```python
from build123d import *

# Parameters (mm, degrees)
SKETCH1_R                       = 90
BOSS_EXTRUDE1_DEPTH             = 2
CUT_EXTRUDE1_DEPTH              = 3
SKETCH5_R                       = 1.75
CUT_EXTRUDE3_DEPTH              = 3
MIRROR2_COPY_1_DEPTH            = 3
MIRROR2_COPY_2_SKETCH_R         = 1.75
MIRROR2_COPY_2_DEPTH            = 3
CUT_EXTRUDE2_DEPTH              = 3
SKETCH6_R                       = 10
CUT_EXTRUDE4_DEPTH              = 3
SKETCH7_R                       = 1.75
CUT_EXTRUDE5_DEPTH              = 3
CIRPATTERN1_COUNT               = 4
CIRPATTERN1_ANGLE               = 36
CIRPATTERN1_THE_OTHER_WAY_COUNT = 4
CIRPATTERN1_THE_OTHER_WAY_ANGLE = 36
SKETCH8_R                       = 1.75
CUT_EXTRUDE6_DEPTH              = 3
SKETCH9_R                       = 1.75
CUT_EXTRUDE7_DEPTH              = 3
CIRPATTERN2_COUNT               = 2
CIRPATTERN2_ANGLE               = 8
CIRPATTERN2_THE_OTHER_WAY_COUNT = 2
CIRPATTERN2_THE_OTHER_WAY_ANGLE = 8
MIRROR3_COPY_1_SKETCH_R         = 1.75
MIRROR3_COPY_1_DEPTH            = 3
MIRROR3_COPY_2_SKETCH_R         = 1.75
MIRROR3_COPY_2_DEPTH            = 3
SKETCH10_R                      = 2
CUT_EXTRUDE8_DEPTH              = 3
LPATTERN1_COUNT                 = 5
LPATTERN1_PITCH                 = 10
LPATTERN1_COPY_1_SKETCH_R       = 2
LPATTERN1_COPY_1_DEPTH          = 3
LPATTERN1_COPY_2_SKETCH_R       = 2
LPATTERN1_COPY_2_DEPTH          = 3
LPATTERN1_COPY_3_SKETCH_R       = 2
LPATTERN1_COPY_3_DEPTH          = 3
LPATTERN1_COPY_4_SKETCH_R       = 2
LPATTERN1_COPY_4_DEPTH          = 3


with BuildPart() as part:
    # Sketch1 → Boss-Extrude1 (new body)
    with BuildSketch(Plane(origin=(0, 0, 0), x_dir=(1, 0, 0), z_dir=(0, 1, 0))):
        Circle(SKETCH1_R)
    extrude(amount=BOSS_EXTRUDE1_DEPTH)

    # Sketch3 → Cut-Extrude1 (cut, through all)
    with BuildSketch(Plane(origin=(0, 2, 0), x_dir=(1, 0, 0), z_dir=(0, 1, 0))):
        Polygon((-106.374227687, 31.753350771), (-80.374227687, 76.786671768), (-49.197313151, 58.786671768), (-75.197313151, 13.753350771), align=None)
    cut_extrude1 = extrude(amount=-CUT_EXTRUDE1_DEPTH, mode=Mode.SUBTRACT)

    # Sketch5 → Cut-Extrude3 (cut, through all)
    with BuildSketch(Plane(origin=(0, 2, 0), x_dir=(1, 0, 0), z_dir=(0, 1, 0))):
        with Locations((-60.537059113, 19.145655616)):
            Circle(SKETCH5_R)
        with Locations((-46.537059113, 43.394366922)):
            Circle(SKETCH5_R)
    cut_extrude3 = extrude(amount=-CUT_EXTRUDE3_DEPTH, mode=Mode.SUBTRACT)

    # Mirror1: Cut-Extrude1, Cut-Extrude3 across plane
    add(cut_extrude1.mirror(Plane.XY), mode=Mode.SUBTRACT)
    add(cut_extrude3.mirror(Plane.XY), mode=Mode.SUBTRACT)

    # Mirror2: Cut-Extrude1, Cut-Extrude3 across plane
    add(cut_extrude1.mirror(Plane(origin=(0, 0, 0), x_dir=(0, 0, 1), z_dir=(1, 0, 0))), mode=Mode.SUBTRACT)
    add(cut_extrude3.mirror(Plane(origin=(0, 0, 0), x_dir=(0, 0, 1), z_dir=(1, 0, 0))), mode=Mode.SUBTRACT)

    # Mirror2 copy 1 sketch → Mirror2 copy 1 (cut, through all)
    with BuildSketch(Plane(origin=(0, 2, 0), x_dir=(-1, 0, 0), z_dir=(0, 1, 0))):
        Polygon((-106.374227687, 31.753350771), (-80.374227687, 76.786671768), (-49.197313151, 58.786671768), (-75.197313151, 13.753350771), align=None)
    extrude(amount=-MIRROR2_COPY_1_DEPTH, mode=Mode.SUBTRACT)

    # Mirror2 copy 2 sketch → Mirror2 copy 2 (cut, through all)
    with BuildSketch(Plane(origin=(0, 2, 0), x_dir=(-1, 0, 0), z_dir=(0, 1, 0))):
        with Locations((-60.537059113, 19.145655616)):
            Circle(MIRROR2_COPY_2_SKETCH_R)
        with Locations((-46.537059113, 43.394366922)):
            Circle(MIRROR2_COPY_2_SKETCH_R)
    extrude(amount=-MIRROR2_COPY_2_DEPTH, mode=Mode.SUBTRACT)

    # Sketch4 → Cut-Extrude2 (cut, through all)
    with BuildSketch(Plane(origin=(0, 2, 0), x_dir=(1, 0, 0), z_dir=(0, 1, 0))):
        with BuildLine():
            Line((-42.5, 79.333158263), (-42.5, 69.333158263))
            ThreePointArc((-42.5, 69.333158263), (0, 55), (42.5, 69.333158263))
            Line((42.5, 69.333158263), (42.5, 79.333158263))
            Line((42.5, 79.333158263), (42.5, 105.809765059))
            Line((42.5, 105.809765059), (-42.5, 105.809765059))
            Line((-42.5, 105.809765059), (-42.5, 79.333158263))
        make_face()
    extrude(amount=-CUT_EXTRUDE2_DEPTH, mode=Mode.SUBTRACT)

    # Sketch6 → Cut-Extrude4 (cut, through all)
    with BuildSketch(Plane(origin=(0, 2, 0), x_dir=(1, 0, 0), z_dir=(0, 1, 0))):
        Circle(SKETCH6_R)
    extrude(amount=-CUT_EXTRUDE4_DEPTH, mode=Mode.SUBTRACT)

    # Sketch7 → Cut-Extrude5 (cut, through all)
    with BuildSketch(Plane.XZ):
        with Locations((0, 86)):
            Circle(SKETCH7_R)
    cut_extrude5 = extrude(amount=-CUT_EXTRUDE5_DEPTH, mode=Mode.SUBTRACT)

    # CirPattern1: Cut-Extrude5 ×4 about axis
    cirpattern1_axis = Axis((0, 0, 0), (0, 1, 0))
    for i in range(1, CIRPATTERN1_COUNT):
        add(cut_extrude5.rotate(cirpattern1_axis, i * CIRPATTERN1_ANGLE / (CIRPATTERN1_COUNT - 1)), mode=Mode.SUBTRACT)

    # CirPattern1 the other way: Cut-Extrude5 ×4 about axis
    cirpattern1_the_other_way_axis = Axis((0, 0, 0), (0, -1, 0))
    for i in range(1, CIRPATTERN1_THE_OTHER_WAY_COUNT):
        add(cut_extrude5.rotate(cirpattern1_the_other_way_axis, i * CIRPATTERN1_THE_OTHER_WAY_ANGLE / (CIRPATTERN1_THE_OTHER_WAY_COUNT - 1)), mode=Mode.SUBTRACT)

    # Sketch8 → Cut-Extrude6 (cut, through all)
    with BuildSketch(Plane(origin=(0, 2, 0), x_dir=(1, 0, 0), z_dir=(0, 1, 0))):
        with Locations((-86, 0)):
            Circle(SKETCH8_R)
    cut_extrude6 = extrude(amount=-CUT_EXTRUDE6_DEPTH, mode=Mode.SUBTRACT)

    # Sketch9 → Cut-Extrude7 (cut, through all)
    with BuildSketch(Plane(origin=(0, 2, 0), x_dir=(1, 0, 0), z_dir=(0, 1, 0))):
        with Locations((-49.706440821, 70.180266036)):
            Circle(SKETCH9_R)
    cut_extrude7 = extrude(amount=-CUT_EXTRUDE7_DEPTH, mode=Mode.SUBTRACT)

    # CirPattern2: Cut-Extrude6 ×2 about axis
    cirpattern2_axis = Axis((0, 2, 0), (0, 1, 0))
    for i in range(1, CIRPATTERN2_COUNT):
        add(cut_extrude6.rotate(cirpattern2_axis, i * CIRPATTERN2_ANGLE / (CIRPATTERN2_COUNT - 1)), mode=Mode.SUBTRACT)

    # CirPattern2 the other way: Cut-Extrude6 ×2 about axis
    cirpattern2_the_other_way_axis = Axis((0, 2, 0), (0, -1, 0))
    for i in range(1, CIRPATTERN2_THE_OTHER_WAY_COUNT):
        add(cut_extrude6.rotate(cirpattern2_the_other_way_axis, i * CIRPATTERN2_THE_OTHER_WAY_ANGLE / (CIRPATTERN2_THE_OTHER_WAY_COUNT - 1)), mode=Mode.SUBTRACT)

    # Mirror3: Cut-Extrude7, Cut-Extrude6 across plane
    add(cut_extrude7.mirror(Plane(origin=(0, 0, 0), x_dir=(0, 0, 1), z_dir=(1, 0, 0))), mode=Mode.SUBTRACT)
    add(cut_extrude6.mirror(Plane(origin=(0, 0, 0), x_dir=(0, 0, 1), z_dir=(1, 0, 0))), mode=Mode.SUBTRACT)

    # Mirror3 copy 1 sketch → Mirror3 copy 1 (cut, through all)
    with BuildSketch(Plane(origin=(0, 2, 0), x_dir=(-0.990268069, 0, -0.139173101), z_dir=(0, 1, 0))):
        with Locations((-86, 0)):
            Circle(MIRROR3_COPY_1_SKETCH_R)
    extrude(amount=-MIRROR3_COPY_1_DEPTH, mode=Mode.SUBTRACT)

    # Mirror3 copy 2 sketch → Mirror3 copy 2 (cut, through all)
    with BuildSketch(Plane(origin=(0, 2, 0), x_dir=(-0.990268069, 0, 0.139173101), z_dir=(0, 1, 0))):
        with Locations((-86, 0)):
            Circle(MIRROR3_COPY_2_SKETCH_R)
    extrude(amount=-MIRROR3_COPY_2_DEPTH, mode=Mode.SUBTRACT)

    # Sketch10 → Cut-Extrude8 (cut, through all)
    with BuildSketch(Plane(origin=(0, 2, 0), x_dir=(1, 0, 0), z_dir=(0, 1, 0))):
        with Locations((14, 50)):
            Circle(SKETCH10_R)
    cut_extrude8 = extrude(amount=-CUT_EXTRUDE8_DEPTH, mode=Mode.SUBTRACT)

    # Mirror4: Cut-Extrude8 across plane
    add(cut_extrude8.mirror(Plane(origin=(0, 0, 0), x_dir=(0, 0, 1), z_dir=(1, 0, 0))), mode=Mode.SUBTRACT)

    # LPattern1: Cut-Extrude8 ×5
    with Locations(*[(0, 0, i * LPATTERN1_PITCH) for i in range(1, LPATTERN1_COUNT)]):
        add(cut_extrude8, mode=Mode.SUBTRACT)

    # LPattern1 copy 1 sketch → LPattern1 copy 1 (cut, through all)
    with BuildSketch(Plane(origin=(0, 2, 10), x_dir=(-1, 0, 0), z_dir=(0, 1, 0))):
        with Locations((14, -50)):
            Circle(LPATTERN1_COPY_1_SKETCH_R)
    extrude(amount=-LPATTERN1_COPY_1_DEPTH, mode=Mode.SUBTRACT)

    # LPattern1 copy 2 sketch → LPattern1 copy 2 (cut, through all)
    with BuildSketch(Plane(origin=(0, 2, 20), x_dir=(-1, 0, 0), z_dir=(0, 1, 0))):
        with Locations((14, -50)):
            Circle(LPATTERN1_COPY_2_SKETCH_R)
    extrude(amount=-LPATTERN1_COPY_2_DEPTH, mode=Mode.SUBTRACT)

    # LPattern1 copy 3 sketch → LPattern1 copy 3 (cut, through all)
    with BuildSketch(Plane(origin=(0, 2, 30), x_dir=(-1, 0, 0), z_dir=(0, 1, 0))):
        with Locations((14, -50)):
            Circle(LPATTERN1_COPY_3_SKETCH_R)
    extrude(amount=-LPATTERN1_COPY_3_DEPTH, mode=Mode.SUBTRACT)

    # LPattern1 copy 4 sketch → LPattern1 copy 4 (cut, through all)
    with BuildSketch(Plane(origin=(0, 2, 40), x_dir=(-1, 0, 0), z_dir=(0, 1, 0))):
        with Locations((14, -50)):
            Circle(LPATTERN1_COPY_4_SKETCH_R)
    extrude(amount=-LPATTERN1_COPY_4_DEPTH, mode=Mode.SUBTRACT)


solid = part.part
```
The listing builds one solid part. Answer for the finished solid, in the listing's coordinates (mm). A direction names the side the tool comes from. Round coordinates to 2 decimals unless told otherwise and drop trailing zeros. Write each loop counter-clockwise with the first axis right and the second up, starting at its lowest first coordinate (ties: lowest second). Pieces come first, ordered by that corner, then holes. Notation, with made-up numbers: (9.25, 27) -> (56.25, 27) arc R28 ccw to (56.25, 62) -> close; hole circle Ø5 at (-5.5, 29.5). An arc over 180 degrees is marked (long way). Write item = value, one per line.
1) Which of the six approach directions +Z, -Z, +X, -X, +Y, -Y give full straight-line access (tool end or side, diameter ignored) to faces 5 (the flat face through (55.37, 1.01, 62.35)), 6 (the flat face through (81.284, 1.014, -17.268)), 7 (the cylindrical face through (-0.946, 0.986, 89.995))?
Check values:
face_5 = +X, +Y, -Y
face_6 = -Z, +Y, -Y
face_7 = +Z, +Y, -Y
2) Straight lines are drawn through the part: line 1 along Z through (x, y) = (0, 1.1); line 2 along Z through (x, y) = (50.5, 1.2); line 3 along X through (y, z) = (1.7, -44.5). For each, find the intervals that lie inside material, in ascending order. Write a range as [from, to].
Check values:
line_1 = [-55, -10], [10, 84.25], [87.75, 90]
line_2 = [-74.5, -71.74], [-68.62, -59.54], [-56.53, 56.53], [59.54, 67.83], [71.32, 74.5]
line_3 = [-57.45, -47.89], [-45.18, 45.18], [47.89, 57.45]
3) Section A-A on x = -14 is taken. Write down the section's boundary in (y, z).
Check values:
outline = (0, -56.41) -> (2, -56.41) -> (2, -52) -> (0, -52) -> close; (0, -48) -> (2, -48) -> (2, -42) -> (0, -42) -> close; (0, -38) -> (2, -38) -> (2, -32) -> (0, -32) -> close; (0, -28) -> (2, -28) -> (2, -22) -> (0, -22) -> close; (0, -18) -> (2, -18) -> (2, -12) -> (0, -12) -> close; (0, -8) -> (2, -8) -> (2, 88.9) -> (0, 88.9) -> close
4) Section B-B on z = 5.5 is taken. Write down the section's boundary in (x, y), plus the area to 3 significant figures.
Check values:
outline = (-89.83, 0) -> (-8.35, 0) -> (-8.35, 2) -> (-89.83, 2) -> close; (8.35, 0) -> (89.83, 0) -> (89.83, 2) -> (8.35, 2) -> close
area = 326 mm²
5) Section C-C on y = 1.3 is taken. Give the number of separate pieces and of enclosed holes in the cut face, plus the area to 3 significant figures.
Check values:
separate_pieces = 1
enclosed_holes = 34
area = 19,000 mm²
6) Section D-D on x = 71 is taken. Write down the section's boundary in (y, z).
Check values:
outline = (0, -21.02) -> (2, -21.02) -> (2, 21.02) -> (0, 21.02) -> close
7) For a pull along X with two mould halves and no side action, classify faces 1 (the flat face through (-55.37, 1.01, 62.35)), 2 (the flat face through (81.284, 1.014, 17.268)), 3 (the flat face through (55.37, 1.01, -62.35)), 4 (the cylindrical face through (14, 1, -38)) as released by +X, released by -X, zero draft, split by the parting line, or undercut.
Check values:
face_1 = released by -X
face_2 = undercut
face_3 = released by +X
face_4 = undercut
8) Given pin 1 (2 mm diameter, centred on x = 50.55, z = 69.58, fed in from +Y); pin 2 (1 mm diameter, centred on x = 67, y = 0.5, fed in from +Z), each flat-ended and moving along its own axis, determine where each tip first touches the part or whether it passes through.
Check values:
pin_1 = through
pin_2 = 28.82
